Model file for the job. Use its own axes, mm. Face numbers are marked on the shaded views. A direction names the side the tool comes from. Round coordinates to 2 decimals unless told otherwise and drop trailing zeros. Loops run counter-clockwise (first coordinate to the right, second up) from the corner with the lowest first, then second, coordinate; pieces in that order, holes last.
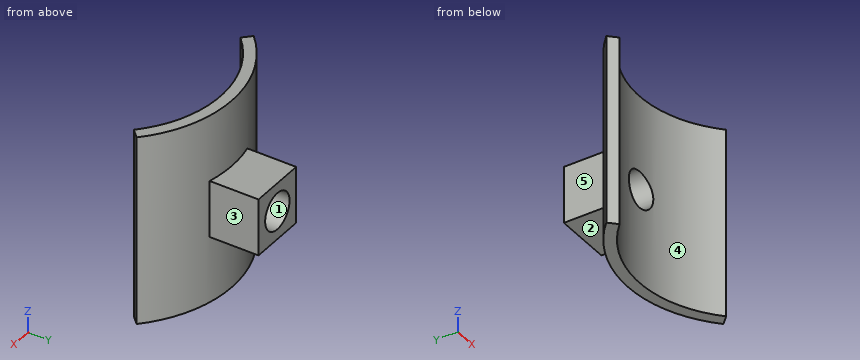
Autodesk Fusion 360 part; units mm, degrees
sketch "Boceto1" plane through (0, 0, 0) normal (0, 0, 1) x (1, 0, 0)
  line L0 (0, 0) -> (23.3345, 23.3345)
  line L1 (0, 0) -> (33, 0) construction
  line L2 (0, 0) -> (-23.3345, 23.3345)
  arc A0 (33, 0) -> (-23.3345, 23.3345) centre (0, 0) ccw
  arc A1 (21.2132, 21.2132) -> (-21.2132, 21.2132) centre (0, 0) ccw
  dimension "d1" = 60
  dimension "d3" = 45
extrude "Extruir1" add sketch "Boceto1" along normal blind 50 contours L0 L2 A0 A1
ref_plane "PlanoDeObra1" through (0, 45, 0) normal (0, 1, 0) x (0, 0, 1)
sketch "Boceto2" plane through (0, 45, 0) normal (0, 1, 0) x (1, 0, 0)
  circle A0 centre (0.0223, -25) radius 4.85
  line L0 (7.5223, -17.5) -> (-7.4777, -17.5)
  line L1 (-7.4777, -17.5) -> (-7.4777, -32.5)
  line L2 (-7.4777, -32.5) -> (7.5223, -32.5)
  line L3 (7.5223, -32.5) -> (7.5223, -17.5)
  line L4 (7.5223, -17.5) -> (-7.4777, -32.5) construction
  line L5 (-7.4777, -17.5) -> (7.5223, -32.5) construction
  point P0 (0.0223, -25)
  dimension "d7" = 9.7
  dimension "d8" = 25
  dimension "d9" = 15
  dimension "d10" = 15
extrude "Extruir2" add sketch "Boceto2" against normal blind 14
extrude "Extruir3" cut sketch "Boceto2" against normal blind 31 contours A0
Q1. Probe line 1 (X direction, y = 37.5, z = 25); line 2 (Y direction, x = 0, z = 14.5); line 3 (X direction, y = 24.75, z = 21). List the from-to ranges inside material, lowest first.
Q2. Slice it at D-D on z = 19.5. Give the cut face in (x, y), plus the area to 3 significant figures.
Q3. Slice it at C-C on y = 43.5. Give the cut face in (x, z), plus the area to 3 significant figures.
Q4. Flat gauge pins, fed straight in: P1, Ø10.5, axis at x = 1, y = 41, coming from the -Z side; P2, Ø6.5, axis at y = 40.5, z = 22.5, coming from the -X side; P3, Ø3, axis at y = 35.5, z = 29, coming from the +X side. Where does each tip first touch, or does it go through?
Q5. Tool access for the marked faces 4 and 5: list every direction of +Z, -Z, +X, -X, +Y, -Y with a clear straight run to the whole face (end or side of a thin tool).
Q6. Slice it at B-B on z = 25. Give the cut face in (x, y).
Q7. Slice it at A-A on y = 24. Give the cut face in (x, z), plus the area to 3 significant figures.
Q8. Pull direction X, two halves, no side cores. Call the marked faces 1, 2 and 3: pulls with the +X half, pulls with the -X half, needs draft (parallel to the pull), parting line crosses it, or undercut.
Reply:
1. line 1: x = -7.48 to -4.83, 4.87 to 7.52
1. line 2: y = 30 to 33
1. line 3: x = -21.83 to -16.95, 16.95 to 21.83
2. outline: (-23.33, 23.33) - (-21.21, 21.21) arc R30 cw to (21.21, 21.21) - (23.33, 23.33) arc R33 ccw to (7.52, 32.13) - (7.52, 45) - (-7.48, 45) - (-7.48, 32.14) arc R33 ccw to start
2. area: 333 mm2
3. outline: (-7.48, 17.5) - (7.52, 17.5) - (7.52, 32.5) - (-7.48, 32.5) - close; hole circle Ø9.7 at (0.02, 25)
3. area: 151 mm2
4. P1: stops at z = 17.5
4. P2: stops at x = -7.48
4. P3: stops at x = 7.52
5. face 4: +Z, -Z, -Y
5. face 5: +Z, -Z, -X, +Y
6. outline: (-23.33, 23.33) - (-21.21, 21.21) arc R30 cw to (-4.83, 29.61) - (-4.83, 45) - (-7.48, 45) - (-7.48, 32.14) arc R33 ccw to start; (4.87, 29.6) arc R30 cw to (21.21, 21.21) - (23.33, 23.33) arc R33 ccw to (7.52, 32.13) - (7.52, 45) - (4.87, 45) - close
7. outline: (-22.65, 0) - (-18, 0) - (-18, 50) - (-22.65, 50) - close; (18, 0) - (22.65, 0) - (22.65, 50) - (18, 50) - close
7. area: 465 mm2
8. face 1: undercut
8. face 2: needs draft
8. face 3: pulls with the +X half
